For this review, take the finished solid that the model builds, in its own axes (mm). Face numbers are marked on the shaded views. A direction names the side the tool comes from. Round coordinates to 2 decimals unless told otherwise and drop trailing zeros. Loops run counter-clockwise (first coordinate to the right, second up) from the corner with the lowest first, then second, coordinate; pieces in that order, holes last. Notation, with made-up numbers: (28, -4.5) -> (72, -4.5) arc R3 cw to (72, 0.5) -> close; hole circle Ø10 at (-38.75, -14.5). An arc over 180 degrees is marked (long way). Write each question's results on one line, items separated by ' | '.
```python
from build123d import *

# Parameters (mm, degrees)
SKETCH_2_R               = 10
CUT_EXTRUDE_1_DEPTH      = 102.323474928
PATTERN_CIRCULAR_1_COUNT = 3
CUT_EXTRUDE_2_DEPTH      = 102.323474928
PATTERN_CIRCULAR_2_COUNT = 8


with BuildPart() as part:
    # Sketch 1 → Revolve 1 (revolve)
    with BuildSketch(Plane.XY, mode=Mode.PRIVATE) as revolve_1_sk:
        Polygon((-3.597374179, 35.5), (-3.597374179, 70), (-14.857768053, 70), (-14.857768053, 33.5), (-21.597374179, 33.5), (-21.597374179, 16), (-8.097374179, 16), (-8.097374179, 21.5), (-4.597374179, 21.5), (-4.597374179, 35.5), align=None)
    revolve(revolve_1_sk.sketch.rotate(Axis((-66.01750547, 0, 0), (1, 0, 0)), 90), axis=Axis((-66.01750547, 0, 0), (1, 0, 0)))

    # Sketch 2 → Cut-Extrude 1 (cut, through all)
    with BuildSketch(Plane(origin=(0, 0, 0), x_dir=(0, 0, -1), z_dir=(1, 0, 0))):
        with Locations((0, 45.357)):
            Circle(SKETCH_2_R)
    cut_extrude_1 = extrude(amount=-CUT_EXTRUDE_1_DEPTH, mode=Mode.SUBTRACT)

    # Pattern Circular 1: Cut-Extrude 1 ×3 about axis
    pattern_circular_1_axis = Axis((0, 0, 0), (1, 0, 0))
    for i in range(1, PATTERN_CIRCULAR_1_COUNT):
        add(cut_extrude_1.rotate(pattern_circular_1_axis, i * 360 / PATTERN_CIRCULAR_1_COUNT), mode=Mode.SUBTRACT)

    # Sketch 3 → Cut-Extrude 2 (cut, through all)
    with BuildSketch(Plane(origin=(0, 0, 0), x_dir=(0, 0, -1), z_dir=(1, 0, 0))):
        with BuildLine():
            Line((3, 15.716233646), (3, 18.761663039))
            ThreePointArc((3, 18.761663039), (0, 19), (-3, 18.761663039))
            Line((-3, 18.761663039), (-3, 15.716233646))
            ThreePointArc((-3, 15.716233646), (0, 16), (3, 15.716233646))
        make_face()
    cut_extrude_2 = extrude(amount=-CUT_EXTRUDE_2_DEPTH, mode=Mode.SUBTRACT)

    # Pattern Circular 2: Cut-Extrude 2 ×8 about axis
    pattern_circular_2_axis = Axis((0, 0, 0), (1, 0, 0))
    for i in range(1, PATTERN_CIRCULAR_2_COUNT):
        add(cut_extrude_2.rotate(pattern_circular_2_axis, i * 360 / PATTERN_CIRCULAR_2_COUNT), mode=Mode.SUBTRACT)


solid = part.part
```
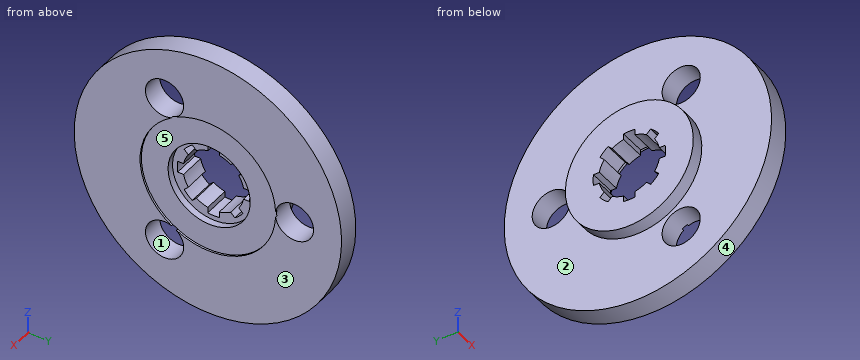
1. Consider section B-B (z = 47). State the section outline as (x, y) points.
Values found:
outline: (-14.86, -51.87) -> (-3.6, -51.87) -> (-3.6, -29.04) -> (-14.86, -29.04) -> close; (-14.86, -16.32) -> (-3.6, -16.32) -> (-3.6, 51.87) -> (-14.86, 51.87) -> close
2. Consider section C-C (z = 26.5). State the section outline as (x, y) points, plus the area to 3 significant figures.
Values found:
outline: (-21.6, -20.49) -> (-14.86, -20.49) -> (-14.86, -64.79) -> (-3.6, -64.79) -> (-3.6, -23.62) -> (-4.6, -23.62) -> (-4.6, 23.62) -> (-3.6, 23.62) -> (-3.6, 64.79) -> (-14.86, 64.79) -> (-14.86, 20.49) -> (-21.6, 20.49) -> close | area: 1,690 mm2
3. Draft analysis for pull direction Z (two halves, no side actions). For the marked faces 3, 4 and 5, state which applies: released by +Z, released by -Z, zero draft, split by the parting line, or undercut.
Values found:
face 3: zero draft | face 4: split by the parting line | face 5: undercut
4. Consider section A-A (y = 0). State the section outline as (x, z) points, plus the area to 3 significant figures.
Values found:
outline: (-21.6, -33.5) -> (-14.86, -33.5) -> (-14.86, -70) -> (-3.6, -70) -> (-3.6, -35.5) -> (-4.6, -35.5) -> (-4.6, -21.5) -> (-8.1, -21.5) -> (-8.1, -19) -> (-21.6, -19) -> close; (-21.6, 19) -> (-8.1, 19) -> (-8.1, 21.5) -> (-4.6, 21.5) -> (-4.6, 35.5) -> (-3.6, 35.5) -> (-3.6, 70) -> (-14.86, 70) -> (-14.86, 33.5) -> (-21.6, 33.5) -> close | area: 1,290 mm2
5. Tool access review of the marked faces 1 and 2: name each direction out of +Z, -Z, +X, -X, +Y, -Y from which nothing blocks a thin tool from reaching the whole face with its end or side.
Values found:
face 1: +X, -X | face 2: -X
6. To check wall thickness, follow probe 1 along Y at (x, z) = (-5.35, 0); probe 2 along Y at (x, z) = (-9, 0); probe 3 along Z at (x, y) = (-9.25, -22). State the ranges of each line that lie inside material, in increasing order.
Values found:
probe 1: y = -70 to -21.5, 21.5 to 35.36, 55.36 to 70 | probe 2: y = -70 to -19, 19 to 35.36, 55.36 to 70 | probe 3: z = -66.45 to -49.26, -29.3 to 29.3, 49.26 to 66.45
7. Consider section D-D (x = -11.25). Give the number of separate pieces and of enclosed holes in the cut face, plus the area to 3 significant figures.
Values found:
separate pieces: 1 | enclosed holes: 4 | area: 13,500 mm2
8. For pin 1 (2.5 mm diameter, centred on x = -17.5, z = -18, fed in from +Y); pin 2 (3.5 mm diameter, centred on x = -15.5, y = 17.5, fed in from -Z); pin 3 (8 mm diameter, centred on x = -16.5, z = -31, fed in from -Y); pin 4 (18 mm diameter, centred on y = 45.357, z = 0, fed in from -X), all flat-tipped, find the tip position at first contact; note any pin that passes through.
Values found:
pin 1: stops at y = 29.01 | pin 2: stops at z = -68.18 | pin 3: stops at y = -64.43 | pin 4: passes through
